CAD build for the part. Positions are in the model's coordinates, mm. Face numbers are marked on the shaded views. Give positions to 0.01 mm unless a question says otherwise; leave off trailing zeros. Loops run counter-clockwise (first coordinate to the right, second up) from the corner with the lowest first, then second, coordinate; pieces in that order, holes last. Notation, with made-up numbers: M 42,72.5 L 76,72.5 A11 ccw 76,76.5 Z; hole C 46,-28.75 d6. An arc over 180 degrees is marked long. Answer as CSV lines item,"result".
```python
from build123d import *

# Parameters (mm, degrees)
F0_W     = 140
F0_H     = 60
F1_DEPTH = 60
F5_R     = 10
F6_DEPTH = 10
F4_R     = 10
F7_DEPTH = 105.8
F3_R     = 10
F8_DEPTH = 10


with BuildPart() as f1:
    # F0 (on Top) → F1 (new body)
    with BuildSketch(Plane.XY):
        Rectangle(F0_W, F0_H)
    extrude(amount=F1_DEPTH)

    # F5 (on face) → F6 (join)
    with BuildSketch(Plane.XY.offset(60)):
        with Locations((38.326033, 0.678791)):
            Circle(F5_R)
    extrude(amount=F6_DEPTH)

    # F4 (on face) → F7 (cut)
    with BuildSketch(Plane.XY.offset(60)):
        Circle(F4_R)
    extrude(amount=-F7_DEPTH, mode=Mode.SUBTRACT)

    # F3 (on face) → F8 (cut)
    with BuildSketch(Plane.XY.offset(60)):
        with Locations((-40.310896, -0.563292)):
            Circle(F3_R)
    extrude(amount=-F8_DEPTH, mode=Mode.SUBTRACT)


solid = f1.part
```
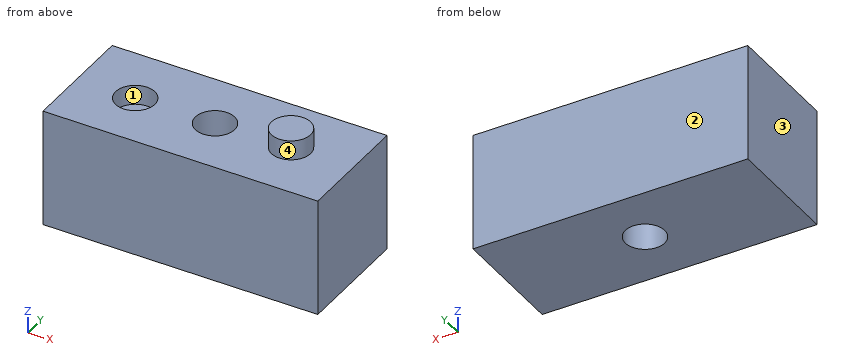
Q1. Cut at B-B (y = -5.5). Write the cut outline in (x, z).
Solution:
outline,"M -70,0 L -8.35,0 L -8.35,60 L -31.61,60 L -31.61,50 L -49.01,50 L -49.01,60 L -70,60 Z; M 8.35,0 L 70,0 L 70,60 L 46.19,60 L 46.19,70 L 30.46,70 L 30.46,60 L 8.35,60 Z"
Q2. Cut at A-A (x = 0). Write the cut outline in (y, z), and give its area (3 significant figures).
Solution:
outline,"M -30,0 L -10,0 L -10,60 L -30,60 Z; M 10,0 L 30,0 L 30,60 L 10,60 Z"
area,"2,400 mm²"
Q3. Wall check: line 1 (X direction, y = 0.5, z = 9.5); line 2 (Y direction, x = 0, z = 36); line 3 (Y direction, x = -40, z = 52). Give the ranges that are in metal, low to high. Write a range as [from, to].
Solution:
line 1,"x = [-70, -9.99], [9.99, 70]"
line 2,"y = [-30, -10], [10, 30]"
line 3,"y = [-30, -10.56], [9.43, 30]"
Q4. Cut at D-D (x = -39). Write the cut outline in (y, z).
Solution:
outline,"M -30,0 L 30,0 L 30,60 L 9.35,60 L 9.35,50 L -10.48,50 L -10.48,60 L -30,60 Z"
Q5. Cut at C-C (z = 24.5). Write the cut outline in (x, y), and give its area (3 significant figures).
Solution:
outline,"M -70,-30 L 70,-30 L 70,30 L -70,30 Z; hole C 0,0 d20"
area,"8,090 mm²"
Q6. Pin check, flat tips, straight feed: P1, Ø6, axis at x = -38.5, y = 3, coming from the +Z side; P2, Ø12, axis at x = -30.5, y = 17, coming from the -Z side; P3, Ø8, axis at x = -27, y = 12.5, coming from the +Z side. Stop position of each tip, or through.
Solution:
P1,"stops at z = 50"
P2,"stops at z = 0"
P3,"stops at z = 60"
Q7. Mould opens along X. For the marked faces 1, 2, 3 and 4 say: released by +X, released by -X, zero draft, split by the parting line, or undercut.
Solution:
face 1,"undercut"
face 2,"zero draft"
face 3,"released by -X"
face 4,"split by the parting line"
